from build123d import *

# Parameters (mm, degrees)
SKETCH_W        = 40
SKETCH_H        = 36
PAD_DEPTH       = 55
SKETCH001_R     = 11.2
SKETCH001_R_2   = 11
POCKET_DEPTH    = 40.001
POCKET001_DEPTH = 4
SKETCH004_R     = 2.2
POCKET002_DEPTH = 51.001
SKETCH005_R     = 3.7
POCKET003_DEPTH = 4.5


with BuildPart() as part:
    # Sketch → Pad (new body)
    with BuildSketch(Plane.XY):
        Rectangle(SKETCH_W, SKETCH_H)
    extrude(amount=PAD_DEPTH)

    # Sketch001 → Pocket (cut, through all)
    with BuildSketch(Plane.YZ.offset(20)):
        with Locations((0, 15)):
            Circle(SKETCH001_R)
        with Locations((0, 40)):
            Circle(SKETCH001_R_2)
    extrude(amount=-POCKET_DEPTH, mode=Mode.SUBTRACT)

    # Sketch002 → Pocket001 (cut)
    with BuildSketch(Plane(origin=(0, 0, 0), x_dir=(1, 0, 0), z_dir=(0, 0, -1))):
        Polygon((2.078461, 9.9), (4.156922, 13.5), (2.078461, 17.1), (-2.078461, 17.1), (-4.156922, 13.5), (-2.078461, 9.9), align=None)
        Polygon((4.156922, -13.5), (2.078461, -9.9), (-2.078461, -9.9), (-4.156922, -13.5), (-2.078461, -17.1), (2.078461, -17.1), align=None)
    extrude(amount=-POCKET001_DEPTH, mode=Mode.SUBTRACT)

    # Sketch004 → Pocket002 (cut, through all)
    with BuildSketch(Plane(origin=(0, 0, 4), x_dir=(1, 0, 0), z_dir=(0, 0, -1))):
        with Locations((0, 13.5)):
            Circle(SKETCH004_R)
        with Locations((0, -13.5)):
            Circle(SKETCH004_R)
    extrude(amount=-POCKET002_DEPTH, mode=Mode.SUBTRACT)

    # Sketch005 → Pocket003 (cut)
    with BuildSketch(Plane.XY.offset(55)):
        with Locations((0, -13.5)):
            Circle(SKETCH005_R)
        with Locations((0, 13.5)):
            Circle(SKETCH005_R)
    extrude(amount=-POCKET003_DEPTH, mode=Mode.SUBTRACT)


solid = part.part
Can you work these out from the model? Positions are in its coordinate system, mm. A direction names the side the tool comes from. Give positions to 0.01 mm unless a question says otherwise; leave off trailing zeros. Write each loop counter-clockwise with the first axis right and the second up, starting at its lowest first coordinate (ties: lowest second). Pieces come first, ordered by that corner, then holes. Notation, with made-up numbers: M 20,18 L 76,18 A16 cw 76,37 Z; hole C 82,80 d5. An arc over 180 degrees is marked long. Answer in a Markdown table with one row per item. Add a question column.
Item 1: Imagine slicing it at A-A, the plane x = 0. State how many separate pieces and enclosed holes the cut face has, plus the area to 3 significant figures.
Item 2: Imagine slicing it at C-C, the plane y = 0. Write out the boundary of the cut face in (x, z).
Item 3: On a 3-axis mill with a long thin cutter (end or side, diameter ignored), from which of +Z, -Z, +X, -X, +Y, -Y can I reach the whole of each face in a straight line? I mean faces 4 (the flat face through (3.132, -15.275, 1.972)), 5 (the flat face through (0, -18, 27)), 6 (the cylindrical face through (-0.48, -9.83, 52.78)). Say none if no direction works.
Item 4: We'd pull the mould along X, two halves only. Please class faces 1 (the flat face through (2, 12, 50.5)), 2 (the flat face through (20, 0, 27)), 3 (the flat face through (0, 0, 55)): released by +X, released by -X, zero draft, split by the parting line, or undercut.
Item 5: Please list where these lines run through material, in increasing order: L1, parallel to Y at x = 0, z = 53; L2, parallel to Y at x = 0, z = 39.5; L3, parallel to Y at x = 0, z = 26.5.
Item 6: For pin 1 Ø20 at (y, z) = (0, 40) entering from +X; pin 2 Ø12 at (x, y) = (0, -13.5) entering from -Z; pin 3 Ø2 at (x, y) = (2, -12.5) entering from +Z, each with a flat end and sliding along its axis, tell me the tip position at first contact or that it passes through.
Item 7: Imagine slicing it at B-B, the plane z = 18.5. Write out the boundary of the cut face in (x, y), plus the area to 3 significant figures.
Item 8: Imagine slicing it at D-D, the plane x = 15. Write out the boundary of the cut face in (y, z), plus the area to 3 significant figures.
Evaluation:
| question | item | result |
|---|---|---|
| 1 | separate pieces | 3 |
| 1 | enclosed holes | 2 |
| 1 | area | 672 mm² |
| 2 | outline | M -20,0 L 20,0 L 20,3.8 L -20,3.8 Z; M -20,26.2 L 20,26.2 L 20,29 L -20,29 Z; M -20,51 L 20,51 L 20,55 L -20,55 Z |
| 3 | face 4 | -Z |
| 3 | face 5 | +Z, -Z, +X, -X, -Y |
| 3 | face 6 | +Z |
| 4 | face 1 | undercut |
| 4 | face 2 | released by +X |
| 4 | face 3 | zero draft |
| 5 | L1 | y = -18 to -17.2, -9.8 to 9.8, 17.2 to 18 |
| 5 | L2 | y = -18 to -15.7, -11.3 to -10.99, 10.99 to 11.3, 15.7 to 18 |
| 5 | L3 | y = -18 to -15.7, -11.3 to 11.3, 15.7 to 18 |
| 6 | pin 1 | passes through |
| 6 | pin 2 | stops at z = 0 |
| 6 | pin 3 | stops at z = 50.5 |
| 7 | outline | M -20,-18 L 20,-18 L 20,-10.64 L -20,-10.64 Z; M -20,10.64 L 20,10.64 L 20,18 L -20,18 Z; hole C 0,-13.5 d4.4; hole C 0,13.5 d4.4 |
| 7 | area | 558 mm² |
| 8 | outline | M -18,0 L 18,0 L 18,55 L -18,55 Z; hole C 0,15 d22.4; hole C 0,40 d22 |
| 8 | area | 1,210 mm² |
